Autodesk Inventor part; units mm, degrees
ref_plane "YZ Plane" through (0, 0, 0) normal (1, 0, 0) x (0, 1, 0)
ref_plane "XZ Plane" through (0, 0, 0) normal (0, 1, 0) x (-1, 0, 0)
ref_plane "XY Plane" through (0, 0, 0) normal (0, 0, 1) x (1, 0, 0)
sketch "Náčrt1" plane through (0, 0, 0) normal (0, 0, 1) x (1, 0, 0)
  line L0 (0, 77) -> (0, -77)
  line L1 (-77, 0) -> (77, 0)
  circle A0 centre (0, 0) radius 55
  dimension "d0" = 110
extrude "Vysunutí1" add sketch "Náčrt1" along normal blind 20
sketch "Náčrt3" plane through (0, 0, 20) normal (0, 0, 1) x (1, 0, 0)
  circle A0 centre (0, 0) radius 52.5
  circle A1 centre (0, 0) radius 51
  dimension "d7" = 105
  dimension "d8" = 102
extrude "Vysunutí3" cut sketch "Náčrt3" against normal blind 3.5
sketch "Náčrt4" plane through (0, 0, 0) normal (0, 0, -1) x (-1, 0, 0)
  line L0 (-8.5, 55) -> (8.5, 55)
  line L1 (8.5, 55) -> (8.5, 15)
  line L2 (8.5, 15) -> (-8.5, 15)
  line L3 (-8.5, 15) -> (-8.5, 55)
  line L4 (0, -77) -> (0, 77)
  line L5 (-77, 0) -> (77, 0)
  circle A0 centre (0, 0) radius 55
  point P0 (0, 55)
  dimension "d11" = 17
  dimension "d12" = 40
extrude "Vysunutí4" cut sketch "Náčrt4" against normal blind 14 contours L0 A0 L3 | A0 L1 L2 L4 | L0 L1 A0 | L4 L2 L3 A0
sketch "Náčrt5" plane through (0, 0, 14) normal (0, 0, -1) x (-1, 0, 0)
  arc A0 (8.5, 54.3392) -> (-8.5, 54.3392) centre (0, 0) ccw
  line L0 (-8.5, 15) -> (-8.5, 54.3392)
  line L1 (8.5, 15) -> (-8.5, 15)
  line L2 (8.5, 54.3392) -> (8.5, 15)
  line L3 (-8.5, 15) -> (8.5, 15)
  line L4 (8.5, 15) -> (8.5, 22)
  line L5 (8.5, 22) -> (-8.5, 22)
  line L6 (-8.5, 22) -> (-8.5, 15)
  point P0 (-8.5, 22)
  dimension "d15" = 7
extrude "Vysunutí5" cut sketch "Náčrt5" against normal through all contours L2 L1 L0 L5
sketch "Náčrt6" plane through (0, 0, 20) normal (0, 0, 1) x (1, 0, 0)
  circle A0 centre (0, 0) radius 43.5
  circle A1 centre (0, 0) radius 42.5
  line L0 (8.5, 15) -> (-8.5, 15)
  line L1 (-8.5, 15) -> (-8.5, 22)
  line L2 (-8.5, 22) -> (8.5, 22)
  line L3 (8.5, 22) -> (8.5, 15)
  circle A2 centre (0, 0) radius 51
  line L4 (0, 77) -> (0, -77)
  dimension "d18" = 87
  dimension "d19" = 85
extrude "Vysunutí6" add sketch "Náčrt6" along normal blind 97 contours A0 L4 A1 | L4 A1 A0
sketch "Náčrt7" plane through (0, 0, 117) normal (0, 0, 1) x (1, 0, 0)
  line L0 (5, 43.5) -> (-5, 43.5)
  line L1 (-5, 43.5) -> (-5, 33.5)
  line L2 (-5, 33.5) -> (5, 33.5)
  line L3 (5, 33.5) -> (5, 43.5)
  circle A0 centre (0, 0) radius 43.5
  line L4 (0, 77) -> (0, -77)
  point P0 (0, 43.5)
  dimension "d22" = 10
  dimension "d23" = 10
extrude "Vysunutí7" cut sketch "Náčrt7" against normal blind 11 contours L3 A0 L0 | A0 L1 L0 | L4 L2 L1 A0 | A0 L3 L2 L4 picked at (-2.7791, 36.7906) picked at (2.7791, 36.7906)
sketch "Náčrt8" plane through (0, 0, 20) normal (0, 0, 1) x (1, 0, 0)
  line L0 (7, -31.1663) -> (-7, -31.1663)
  line L1 (-7, -31.1663) -> (-7, -23.1663)
  line L2 (-7, -23.1663) -> (7, -23.1663)
  line L3 (7, -23.1663) -> (7, -31.1663)
  line L4 (0, 77) -> (0, -77)
  line L5 (-77, 0) -> (77, 0)
  line L6 (16.5, -39.1663) -> (-16.5, -39.1663)
  line L7 (-16.5, -39.1663) -> (-16.5, -31.1663)
  line L8 (-16.5, -31.1663) -> (16.5, -31.1663)
  line L9 (16.5, -31.1663) -> (16.5, -39.1663)
  arc A0 (-5, 42.2049) -> (5, 42.2049) centre (0, 0) ccw
  point P0 (0, -39.1663)
  point P1 (0, -31.1663)
  point P2 (0, -42.5)
  point P3 (-42.5, 0)
  point P4 (0, -23.1663)
  point P5 (42.5, 0)
  point P6 (7, -31.1663)
  dimension "d26" = 33
  dimension "d27" = 8
  dimension "d28" = 14
  dimension "d29" = 8
extrude "Vysunutí8" add sketch "Náčrt8" along normal blind 32 contours L0 L4 L2 L3 | L0 L1 L2 L4
properties part number "krabička"
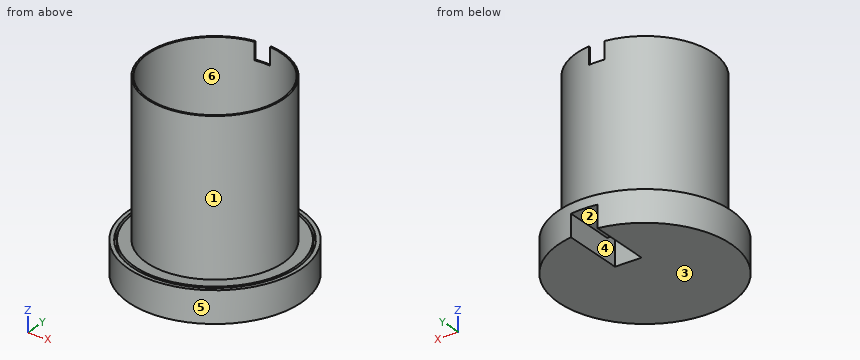
Here's how the part is built. I have some questions about the finished solid (model axes, mm). Face numbers are marked on the shaded views. A direction names the side the tool comes from. Coordinates: 2 decimals unless noted, no trailing zeros. Loops run counter-clockwise (first coordinate to the right, second up) from the corner with the lowest first, then second, coordinate; pieces in that order, holes last.
1. Imagine slicing it at A-A, the plane z = 41. Please give me the cut outline in (x, y), and give its area (3 significant figures).
2. Imagine slicing it at B-B, the plane x = 0. Please give me the cut outline in (y, z).
3. For the marked faces 5 and 6, which set-ups out of +Z, -Z, +X, -X, +Y, -Y let a thin tool reach every point of the face, with its end or its side?
4. For P1, Ø6.5, axis at x = 3.5, y = -28, coming from the +Z side; P2, Ø5, axis at y = -34.5, z = 29, coming from the +X side; P3, Ø4, axis at y = -26, z = 36.5, coming from the -X side, each with a flat end and sliding along its axis, tell me the tip position at first contact or that it passes through.
5. Imagine slicing it at C-C, the plane y = 0. Please give me the cut outline in (x, z).
6. I need wall thicknesses on L1, parallel to Y at x = 0, z = 17.5; L2, parallel to Y at x = 0, z = 86. Which ranges of each line are inside material? Lowest first, please.
7. Imagine slicing it at D-D, the plane z = 90.5. Please give me the cut outline in (x, y), and give its area (3 significant figures).
8. If we mould it in two halves opening along X, with no side actions, what happens to the marked faces 1, 2, 3 and 4? For each: pulls with the +X half, pulls with the -X half, needs draft (parallel to the pull), parting line crosses it, or undercut.
Taken from the geometry:
1. outline: circle Ø87 at (0, 0); (-7, -31.17) - (7, -31.17) - (7, -23.17) - (-7, -23.17) - close; hole circle Ø85 at (0, 0)
1. area: 382 mm2
2. outline: (-55, 0) - (15, 0) - (15, 20) - (-23.17, 20) - (-23.17, 52) - (-31.17, 52) - (-31.17, 20) - (-42.5, 20) - (-42.5, 117) - (-43.5, 117) - (-43.5, 20) - (-51, 20) - (-51, 16.5) - (-52.5, 16.5) - (-52.5, 20) - (-55, 20) - close; (22, 14) - (55, 14) - (55, 20) - (52.5, 20) - (52.5, 16.5) - (51, 16.5) - (51, 20) - (43.5, 20) - (43.5, 106) - (42.5, 106) - (42.5, 20) - (22, 20) - close
3. face 5: +Z, -Z
3. face 6: +Z
4. P1: stops at z = 52
4. P2: stops at x = 29.47
4. P3: stops at x = -36.28
5. outline: (-55, 0) - (55, 0) - (55, 20) - (52.5, 20) - (52.5, 16.5) - (51, 16.5) - (51, 20) - (43.5, 20) - (43.5, 117) - (42.5, 117) - (42.5, 20) - (-42.5, 20) - (-42.5, 117) - (-43.5, 117) - (-43.5, 20) - (-51, 20) - (-51, 16.5) - (-52.5, 16.5) - (-52.5, 20) - (-55, 20) - close
6. L1: y = -55 to -52.5, -51 to 15, 22 to 51, 52.5 to 55
6. L2: y = -43.5 to -42.5, 42.5 to 43.5
7. outline: circle Ø87 at (0, 0); hole circle Ø85 at (0, 0)
7. area: 270 mm2
8. face 1: parting line crosses it
8. face 2: undercut
8. face 3: needs draft
8. face 4: undercut
